Work out the finished part from the listing and answer in its coordinate system (mm). Face numbers are marked on the shaded views. Coordinates: 2 decimals unless noted, no trailing zeros. Write each loop counter-clockwise with the first axis right and the second up, starting at its lowest first coordinate (ties: lowest second). Pieces come first, ordered by that corner, then holes. Notation, with made-up numbers: (33, 71) - (46, 71) arc R29 cw to (46, 107) - close; hole circle Ø5 at (72.25, 30.25). An arc over 180 degrees is marked (long way). One line per item, written item: value.
```python
from build123d import *

# Parameters (mm, degrees)
SKETCH2_R          = 2.55
CUT_EXTRUDE1_DEPTH = 10


with BuildPart() as part:
    # Sketch1 → Revolve1 (revolve)
    with BuildSketch(Plane.XY, mode=Mode.PRIVATE) as revolve1_sk:
        Polygon((0, 0), (0, 10), (3, 10), (3, 7.5), (57.5, 7.5), (57.5, 0), align=None)
    revolve(revolve1_sk.sketch.rotate(Axis((0, 0, 0), (-1, 0, 0)), 90), axis=Axis((0, 0, 0), (-1, 0, 0)))

    # Sketch2 → Cut-Extrude1 (cut)
    with BuildSketch(Plane(origin=(57.5, 0, 0), x_dir=(0, 0, -1), z_dir=(1, 0, 0))):
        Circle(SKETCH2_R)
    extrude(amount=-CUT_EXTRUDE1_DEPTH, mode=Mode.SUBTRACT)


solid = part.part
```
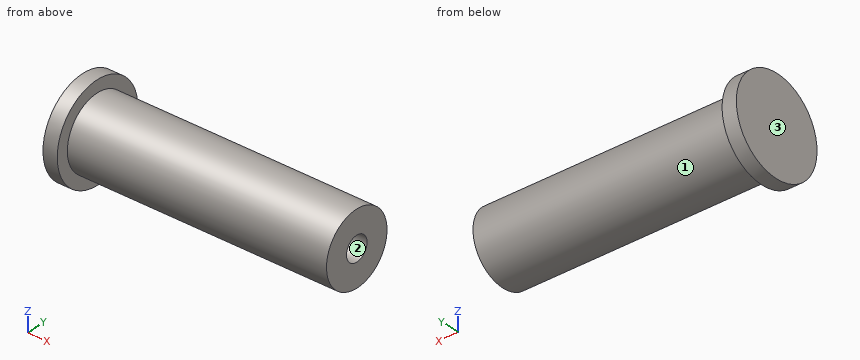
Item 1: Section A-A, the plane z = 0 is taken. Determine the outline of the cut face in (x, y).
Evaluation:
outline: (0, -10) - (3, -10) - (3, -7.5) - (57.5, -7.5) - (57.5, -2.55) - (47.5, -2.55) - (47.5, 2.55) - (57.5, 2.55) - (57.5, 7.5) - (3, 7.5) - (3, 10) - (0, 10) - close
Item 2: Section D-D, the plane z = 6.5 is taken. Determine the outline of the cut face in (x, y).
Evaluation:
outline: (0, -7.6) - (3, -7.6) - (3, -3.74) - (57.5, -3.74) - (57.5, 3.74) - (3, 3.74) - (3, 7.6) - (0, 7.6) - close
Item 3: Section C-C, the plane x = 53.5 is taken. Determine the outline of the cut face in (y, z).
Evaluation:
outline: circle Ø15 at (0, 0); hole circle Ø5.1 at (0, 0)
Item 4: Determine the mould class of the marked faces 1, 2 and 3 for opening direction Z: +Z half, -Z half, draft (parallel to the pull), parting line (faces both ways), or undercut.
Evaluation:
face 1: parting line
face 2: undercut
face 3: draft
Item 5: Given pin 1 (4.5 mm diameter, centred on y = 0, z = 0, fed in from +X); pin 2 (6 mm diameter, centred on x = 18, z = -6, fed in from -Y); pin 3 (1.5 mm diameter, centred on x = 24, y = -3.5, fed in from +Z), each flat-ended and moving along its own axis, determine where each tip first touches the part or whether it passes through.
Evaluation:
pin 1: stops at x = 47.5
pin 2: stops at y = -6.87
pin 3: stops at z = 6.98
Item 6: Section B-B, the plane y = -4.25 is taken. Determine the outline of the cut face in (x, z).
Evaluation:
outline: (0, -9.05) - (3, -9.05) - (3, -6.18) - (57.5, -6.18) - (57.5, 6.18) - (3, 6.18) - (3, 9.05) - (0, 9.05) - close
Item 7: Consider probe 1 along Y at (x, z) = (53.25, 0); probe 2 along X at (y, z) = (-3.25, -7.75); probe 3 along X at (y, z) = (0, 2.25). Determine where each line is inside the solid, lowest interval first.
Evaluation:
probe 1: y = -7.5 to -2.55, 2.55 to 7.5
probe 2: x = 0 to 3
probe 3: x = 0 to 47.5
